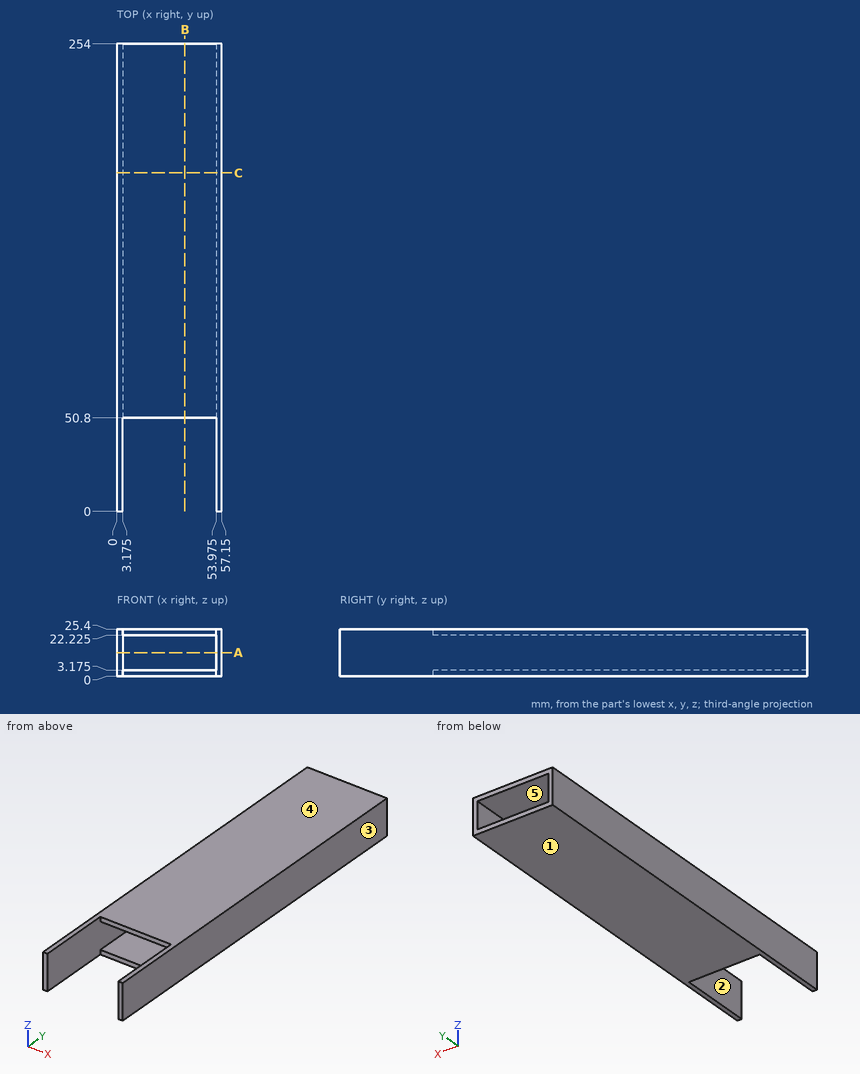
Can you work these out from the drawing? Everything is in mm from the part's minimum corner. A direction names the side the tool comes from. Round coordinates to 2 decimals unless told otherwise and drop trailing zeros. Loops run counter-clockwise (first coordinate to the right, second up) from the corner with the lowest first, then second, coordinate; pieces in that order, holes last.
1. If we section it at A-A on z = 12.75: Write out the boundary of the cut face in (x, y) (3 decimals).
Answer list:
outline: (0, 0) - (3.175, 0) - (3.175, 254) - (0, 254) - close; (53.975, 0) - (57.15, 0) - (57.15, 254) - (53.975, 254) - close
2. If I drill on line 1 along Z through (x, y) = (51.5, 239.5) (3 decimals); line 2 along X through (y, z) = (30, 17) (3 decimals); line 3 along Y through (x, z) = (26, 24), over which ranges is the centre line in solid material (lowest first)?
Answer list:
line 1: z = 0 to 3.175, 22.225 to 25.4
line 2: x = 0 to 3.175, 53.975 to 57.15
line 3: y = 50.8 to 254
3. If we section it at C-C on y = 184: Write out the boundary of the cut face in (x, z) (3 decimals), plus the area to 3 significant figures.
Answer list:
outline: (0, 0) - (57.15, 0) - (57.15, 25.4) - (0, 25.4) - close; hole (3.175, 3.175) - (53.975, 3.175) - (53.975, 22.225) - (3.175, 22.225) - close
area: 484 mm2
4. For P1, Ø3.5, axis at x = 18, z = 1, coming from the -Y side, with a flat end and sliding along its axis, tell me the tip position at first contact or that it passes through.
Answer list:
P1: stops at y = 50.8
5. Which directions (+Z, -Z, +X, -X, +Y, -Y) give clear straight access to the entire face, cutting with the end or side of a thin tool? Please do the marked faces 4 and 5.
Answer list:
face 4: +Z, +X, -X, +Y, -Y
face 5: +Y, -Y
6. We'd pull the mould along X, two halves only. Please class the marked faces 1, 2 and 3: +X half, -X half, draft (parallel to the pull), parting line (faces both ways), or undercut.
Answer list:
face 1: draft
face 2: undercut
face 3: +X half
7. If we section it at B-B on x = 37: Write out the boundary of the cut face in (y, z) (3 decimals), plus the area to 3 significant figures.
Answer list:
outline: (50.8, 0) - (254, 0) - (254, 3.175) - (50.8, 3.175) - close; (50.8, 22.225) - (254, 22.225) - (254, 25.4) - (50.8, 25.4) - close
area: 1,290 mm2
